Geometry check sheet. Reference: the model listing, model coordinates, mm. A direction names the side the tool comes from. Coordinates: 2 decimals unless noted, no trailing zeros. Write each loop counter-clockwise with the first axis right and the second up, starting at its lowest first coordinate (ties: lowest second). Pieces come first, ordered by that corner, then holes. Notation, with made-up numbers: M 12,14.5 L 37,14.5 A20 ccw 37,27.5 Z; hole C 22.25,63 d3. An arc over 180 degrees is marked long. Put each result on its own line as item: value. Start each with the question number.
1) Cross-section at B-B on x = -25.4. Record the cut outline in (y, z), plus the area to 3 significant figures.
2) Cross-section at A-A on z = 0. Record the cut outline in (x, y) (3 decimals), plus the area to 3 significant figures.
3) Gauge pin test, flat ends, axial feed: pin 1 (24.5 mm diameter, centred on x = 11.5, z = 4, fed in from -Y); pin 2 (2 mm diameter, centred on x = 7, y = -16.5, fed in from +Z); pin 3 (12 mm diameter, centred on y = -7.5, z = -23, fed in from +X); pin 4 (5 mm diameter, centred on x = 24, y = -14.5, fed in from +Z). Record the tip position at first contact, or that the pin passes through.
4) Cross-section at D-D on x = 0. Record the cut outline in (y, z) (3 decimals), plus the area to 3 significant figures.
5) Cross-section at C-C on y = -17.5. Record the cut outline in (x, z) (3 decimals).
6) Set-up check for faces 1 (the cylindrical face through (-5.264, -16.008, -23.705)), 2 (the cylindrical face through (37.336, 2.504, -37.376)): record each of +Z, -Z, +X, -X, +Y, -Y from which the full face is reachable in a straight line by a thin tool's end or side.
7) Scan lines: line 1 along X through (y, z) = (3, 25); line 2 along Z through (x, y) = (25.4, 2.65); line 3 along Z through (x, y) = (0, -15) (3 decimals). Record each from-to range of solid material in increasing order.
8) Mould release check, pull along Z, two halves, no side actions. Record for faces 3 (the cylindrical face through (-28.42, 2.5, 27.72)), 4 (the flat face through (1, 5.08, -1)), 5 (the cylindrical face through (37.376, 2.504, 37.336)): released by +Z, released by -Z, zero draft, split by the parting line, or undercut.
from build123d import *

# Parameters (mm, degrees)
SKETCH2_R           = 3.81
BOSS_EXTRUDE1_DEPTH = 5.08
SKETCH3_R           = 28.575
BOSS_EXTRUDE2_DEPTH = 25.4
SKETCH4_R           = 24.2824
CUT_EXTRUDE1_DEPTH  = 19.05


with BuildPart() as part:
    # Sketch2 → Boss-Extrude1 (new body)
    with BuildSketch(Plane(origin=(0, 0, 0), x_dir=(1, 0, 0), z_dir=(0, 1, 0))):
        with BuildLine():
            Line((-35.56, 38.1), (35.56, 38.1))
            ThreePointArc((35.56, 38.1), (37.356051224, 37.356051224), (38.1, 35.56))
            Line((38.1, 35.56), (38.1, -35.56))
            ThreePointArc((38.1, -35.56), (37.356051224, -37.356051224), (35.56, -38.1))
            Line((35.56, -38.1), (-35.56, -38.1))
            ThreePointArc((-35.56, -38.1), (-37.356051224, -37.356051224), (-38.1, -35.56))
            Line((-38.1, -35.56), (-38.1, 35.56))
            ThreePointArc((-38.1, 35.56), (-37.356051224, 37.356051224), (-35.56, 38.1))
        make_face()
        with Locations((-25.4, 25.4)):
            Circle(SKETCH2_R, mode=Mode.SUBTRACT)
        with Locations((25.4, 25.4)):
            Circle(SKETCH2_R, mode=Mode.SUBTRACT)
        with Locations((25.4, -25.4)):
            Circle(SKETCH2_R, mode=Mode.SUBTRACT)
        with Locations((-25.4, -25.4)):
            Circle(SKETCH2_R, mode=Mode.SUBTRACT)
    extrude(amount=BOSS_EXTRUDE1_DEPTH)

    # Sketch3 → Boss-Extrude2 (add)
    with BuildSketch(Plane.XZ):
        Circle(SKETCH3_R)
    extrude(amount=BOSS_EXTRUDE2_DEPTH)

    # Sketch4 → Cut-Extrude1 (cut)
    with BuildSketch(Plane.XZ.offset(25.4)):
        Circle(SKETCH4_R)
    extrude(amount=-CUT_EXTRUDE1_DEPTH, mode=Mode.SUBTRACT)


solid = part.part
Answer key:
1. outline: M -25.4,-13.09 L 0,-13.09 L 0,-21.59 L 5.08,-21.59 L 5.08,21.59 L 0,21.59 L 0,13.09 L -25.4,13.09 Z; M 0,-38.1 L 5.08,-38.1 L 5.08,-29.21 L 0,-29.21 Z; M 0,29.21 L 5.08,29.21 L 5.08,38.1 L 0,38.1 Z
1. area: 975 mm²
2. outline: M -38.1,0 L -28.575,0 L -28.575,-25.4 L -24.282,-25.4 L -24.282,-6.35 L 24.282,-6.35 L 24.282,-25.4 L 28.575,-25.4 L 28.575,0 L 38.1,0 L 38.1,5.08 L -38.1,5.08 Z
2. area: 914 mm²
3. pin 1: stops at y = -25.4
3. pin 2: stops at z = 27.94
3. pin 3: stops at x = 22.97
3. pin 4: stops at z = 18.82
4. outline: M -25.4,-28.575 L 0,-28.575 L 0,-38.1 L 5.08,-38.1 L 5.08,38.1 L 0,38.1 L 0,28.575 L -25.4,28.575 L -25.4,24.282 L -6.35,24.282 L -6.35,-24.282 L -25.4,-24.282 Z
4. area: 914 mm²
5. outline: C 0,0 d57.15; hole C 0,0 d48.565
6. face 1: -Y
6. face 2: -Z, +X, +Y, -Y
7. line 1: x = -38.1 to -29.19, -21.61 to 21.61, 29.19 to 38.1
7. line 2: z = -38.1 to -29.21, -21.59 to 21.59, 29.21 to 38.1
7. line 3: z = -28.575 to -24.282, 24.282 to 28.575
8. face 3: undercut
8. face 4: zero draft
8. face 5: released by +Z
